The listing builds one solid part. Answer for the finished solid, in the listing's coordinates (mm). A direction names the side the tool comes from. Give positions to 0.01 mm unless a question says otherwise; leave off trailing zeros. Write each loop counter-clockwise with the first axis right and the second up, starting at its lowest first coordinate (ties: lowest second). Pieces come first, ordered by that corner, then holes. Notation, with made-up numbers: (82, 73.5) - (121, 73.5) arc R17 cw to (121, 104.5) - close; hole circle Ø11 at (58.25, 82). An arc over 180 degrees is marked (long way). Return JSON: item names as keys, results as strings.
from build123d import *

# Parameters (mm, degrees)
SKETCH_1_W            = 27.8
SKETCH_1_H            = 24.2
EXTRUDE_1_DEPTH       = 5
SKETCH_5_R            = 1.4
EXTRUDE_5_DEPTH       = 8
SKETCH_8_W            = 1.5
SKETCH_8_H            = 34.2
CUT_EXTRUDE_1_DEPTH   = 30
EXTRUDE_11_DEPTH      = 10
EXTRUDE_11_DEPTH_BACK = 10
EXTRUDE_12_DEPTH      = 3.9


with BuildPart() as part:
    # 草图1 → 凸台-拉伸1 (new body)
    with BuildSketch(Plane.XY):
        Rectangle(SKETCH_1_W, SKETCH_1_H)
    extrude(amount=EXTRUDE_1_DEPTH)

    # 草图5 → 凸台-拉伸5 (add)
    # profile 1 of 2: a face of its own
    with BuildSketch(Plane.ZY.offset(13.9)):
        Polygon((-11.5, -11.168960062), (-12.967909623, -11.168960062), (-13.608884892, -11.809935331), (-13.608884892, -17.1), (-11.5, -17.1), (5, -17.1), (5, -12.1), (0, -12.1), (-7.82761802, -12.1), (-10.28681363, -11.168960062), align=None)
        with Locations((-11.5, -13.1)):
            Circle(SKETCH_5_R, mode=Mode.SUBTRACT)
    # profile 2 of 2: a face of its own
    with BuildSketch(Plane.ZY.offset(13.9)):
        Polygon((5, 12.1), (5, 17.1), (-11.5, 17.1), (-13.608884892, 17.1), (-13.608884892, 11.809935331), (-12.967909623, 11.168960062), (-11.5, 11.168960062), (-10.28681363, 11.168960062), (-7.82761802, 12.1), (0, 12.1), align=None)
        with Locations((-11.5, 13.1)):
            Circle(SKETCH_5_R, mode=Mode.SUBTRACT)
    extrude_5 = extrude(amount=-EXTRUDE_5_DEPTH)

    # 镜向1: 凸台-拉伸5 across plane
    add(extrude_5.mirror(Plane(origin=(0, 0, 0), x_dir=(0, 0, 1), z_dir=(1, 0, 0))))

    # 草图8 → 切除-拉伸1 (cut)
    with BuildSketch(Plane(origin=(13.9, 0, 0), x_dir=(0, 0, -1), z_dir=(1, 0, 0))):
        with Locations((-4.25, 0)):
            Rectangle(SKETCH_8_W, SKETCH_8_H)
    extrude(amount=-CUT_EXTRUDE_1_DEPTH, mode=Mode.SUBTRACT)

    # 草图10 → 凸台-拉伸11 (add, two sides: drawn at the far end of the back side and taken through both)
    with BuildSketch(Plane(origin=(0, 0, 0), x_dir=(0, 0, -1), z_dir=(1, 0, 0)).offset(-EXTRUDE_11_DEPTH_BACK)):
        Polygon((-3.5, -7), (-13.34807753, -5.263518223), (-13.34807753, 5.263518223), (-3.5, 7), align=None)
        Polygon((-3.5, 16.591331578), (-3.5, 7), (-5.191210538, 16.591331578), align=None)
        Polygon((-5.191210538, -16.591331578), (-3.5, -16.591331578), (-3.5, -7), align=None)
    extrude(amount=EXTRUDE_11_DEPTH + EXTRUDE_11_DEPTH_BACK)

    # 草图11 → 凸台-拉伸12 (add)
    with BuildSketch(Plane.ZY.offset(10)):
        with BuildLine():
            Line((5.191210538, 16.591331578), (4.489460182, 12.611507539))
            Line((4.489460182, 12.611507539), (13.800354116, 12.611507539))
            ThreePointArc((13.800354116, 12.611507539), (15.343887855, 13.227011755), (16.040354116, 14.735745196))
            Line((16.040354116, 14.735745196), (16.040354116, 14.973578462))
            ThreePointArc((16.040354116, 14.973578462), (15.343887855, 16.482311902), (13.800354116, 17.097816118))
            Line((13.800354116, 17.097816118), (3.5, 17.097816118))
            Line((3.5, 17.097816118), (3.5, 16.591331578))
            Line((3.5, 16.591331578), (5.191210538, 16.591331578))
        make_face()
        with BuildLine():
            Line((3.5, -17.097816118), (13.800354116, -17.097816118))
            ThreePointArc((13.800354116, -17.097816118), (16.043508405, -14.854661829), (13.800354116, -12.611507539))
            Line((13.800354116, -12.611507539), (3.5, -12.611507539))
            Line((3.5, -12.611507539), (3.5, -17.097816118))
        make_face()
        Polygon((3.5, 16.591331578), (3.5, 12.611507539), (4.489460182, 12.611507539), (5.191210538, 16.591331578), align=None)
    extrude_12 = extrude(amount=EXTRUDE_12_DEPTH)

    # 镜向3: 凸台-拉伸12 across plane
    add(extrude_12.mirror(Plane(origin=(0, 0, 0), x_dir=(0, 0, 1), z_dir=(1, 0, 0))))


solid = part.part
Item 1: The mould has two halves that part along Y. Classify faces 1 (the face through (10, 11.169, -12)), 2 (the face through (-13.9, -1, 1)), 3 (the face through (0, -16.591, 4)), 4 (the face through (12, 17.098, 9)): +Y half, -Y half, draft (parallel to the pull), parting line (faces both ways), or undercut.
Answer below:
{"face 1": "undercut", "face 2": "draft", "face 3": "-Y half", "face 4": "+Y half"}
Item 2: For faces 5 (the face through (-10, -11, 4)), 6 (the face through (0, 12.1, 2)), 7 (the face through (-0.14, 11.729, 4.334)), 8 (the face through (10, 12.1, -4)), determine the directions among +Z, -Z, +X, -X, +Y, -Y from which every point of the face is accessible in a straight line to the end or side of a thin tool.
Answer below:
{"face 5": "+Z, -X", "face 6": "-Z, +Y", "face 7": "+Z", "face 8": "+X, -X"}
Item 3: A cutting plane is placed at C-C on x = -0.5. Determine the outline of the cut face in (y, z).
Answer below:
{"outline": "(-16.59, 3.5) - (-12.1, 3.5) - (-12.1, 0) - (12.1, 0) - (12.1, 3.5) - (16.59, 3.5) - (16.59, 5.19) - (7, 3.5) - (5.26, 13.35) - (-5.26, 13.35) - (-7, 3.5) - (-16.59, 5.19) - close"}
Item 4: A cutting plane is placed at A-A on z = -11.5. Give the number of separate pieces and of enclosed holes in the cut face, then the cut area to 3 significant figures.
Answer below:
{"separate pieces": "8", "enclosed holes": "0", "area": "100 mm²"}
Item 5: A cutting plane is placed at D-D on z = 1. Determine the outline of the cut face in (x, y), then the cut area to 3 significant figures.
Answer below:
{"outline": "(-13.9, -17.1) - (-5.9, -17.1) - (-5.9, -12.1) - (5.9, -12.1) - (5.9, -17.1) - (13.9, -17.1) - (13.9, 17.1) - (5.9, 17.1) - (5.9, 12.1) - (-5.9, 12.1) - (-5.9, 17.1) - (-13.9, 17.1) - close", "area": "833 mm²"}
Item 6: Flat-ended cylindrical pins translate along their axes: P1, Ø5, axis at x = 10.5, y = 3, coming from the -Z side; P2, Ø2, axis at x = -12.5, y = -0.5, coming from the +Z side; P3, Ø0.5, axis at y = -10.5, z = 4, coming from the -X side; P4, Ø8, axis at x = -5, z = 6, coming from the -Y side. Find the tip coordinate at first contact, or state that the pin passes through.
Answer below:
{"P1": "stops at z = 0", "P2": "stops at z = 3.5", "P3": "stops at x = -10", "P4": "stops at y = -17.1"}
Item 7: Consider L1, parallel to Y at x = -9.75, z = -11.5; L2, parallel to X at y = -14, z = 7.75; L3, parallel to Y at x = 6, z = -1. Determine where each line is inside the solid, lowest interval first.
Answer below:
{"L1": "y = -17.1 to -14.5, -11.7 to -11.17, 11.17 to 11.7, 14.5 to 17.1", "L2": "x = -13.9 to -10, 10 to 13.9", "L3": "y = -17.1 to -12.1, 12.1 to 17.1"}
Item 8: A cutting plane is placed at B-B on y = 13.1. Determine the outline of the cut face in (x, z), then the cut area to 3 significant figures.
Answer below:
{"outline": "(-13.9, -13.61) - (-5.9, -13.61) - (-5.9, -12.9) - (-13.9, -12.9) - close; (-13.9, -10.1) - (-5.9, -10.1) - (-5.9, 3.5) - (5.9, 3.5) - (5.9, -10.1) - (13.9, -10.1) - (13.9, 15.2) - (10, 15.2) - (10, 4.58) - (-10, 4.58) - (-10, 15.2) - (-13.9, 15.2) - close; (5.9, -13.61) - (13.9, -13.61) - (13.9, -12.9) - (5.9, -12.9) - close", "area": "342 mm²"}
